from build123d import *

# Parameters (mm, degrees)
SKETCH1_W                      = 330.2
SKETCH1_H                      = 196.85
BOSS_EXTRUDE1_DEPTH            = 11.1125
SKETCH3_W                      = 317.5
SKETCH3_H                      = 184.15
CUT_EXTRUDE1_DEPTH             = 193.533057632
FILLET1_R                      = 6.35
SKETCH4_W                      = 6.35
SKETCH4_H                      = 11.1125
BOSS_EXTRUDE2_DEPTH            = 184.15
FILLET2_R                      = 6.35
F_8_CLEARANCE_HOLE1_REACH      = 346.736
F_8_CLEARANCE_HOLE1_BORE_R     = 2.2479
F_4_40_TAPPED_HOLE1_AT_2_COUNT = 2
F_4_40_TAPPED_HOLE1_AT_2_PITCH = 57.15
F_4_40_TAPPED_HOLE1_AT_3_COUNT = 2
F_4_40_TAPPED_HOLE1_AT_3_PITCH = 117.475
F_4_40_TAPPED_HOLE1_AT_4_COUNT = 2
F_4_40_TAPPED_HOLE1_AT_4_PITCH = 187.325
F_4_40_TAPPED_HOLE1_AT_5_COUNT = 2
F_4_40_TAPPED_HOLE1_AT_5_PITCH = 247.65
F_4_40_TAPPED_HOLE1_AT_6_COUNT = 2
F_4_40_TAPPED_HOLE1_AT_6_PITCH = 317.5
F_4_40_TAPPED_HOLE2_AT_2_COUNT = 2
F_4_40_TAPPED_HOLE2_AT_2_PITCH = 95.25
LPATTERN1_COUNT                = 2
LPATTERN1_PITCH                = 120.015
CUT_EXTRUDE2_REACH             = 346.736
SKETCH13_W                     = 22.225
SKETCH13_H                     = 5.08


with BuildPart() as part:
    # Sketch1 → Boss-Extrude1 (new body)
    with BuildSketch(Plane(origin=(0, 0, 0), x_dir=(1, 0, 0), z_dir=(0, 1, 0))):
        Rectangle(SKETCH1_W, SKETCH1_H)
    extrude(amount=BOSS_EXTRUDE1_DEPTH)

    # Sketch3 → Cut-Extrude1 (cut, through all)
    with BuildSketch(Plane(origin=(0, 11.1125, 0), x_dir=(1, 0, 0), z_dir=(0, 1, 0))):
        Rectangle(SKETCH3_W, SKETCH3_H)
    extrude(amount=-CUT_EXTRUDE1_DEPTH, mode=Mode.SUBTRACT)

    # Fillet1
    fillet1_edges = [part.edges().sort_by_distance(p)[0] for p in [
        (158.75, 5.55625, -92.075),
        (158.75, 5.55625, 92.075),
        (-158.75, 5.55625, 92.075),
        (-158.75, 5.55625, -92.075),
        (165.1, 5.55625, 98.425),
        (-165.1, 5.55625, 98.425),
        (-165.1, 5.55625, -98.425),
        (165.1, 5.55625, -98.425),
    ]]
    fillet(fillet1_edges, radius=FILLET1_R)

    # Sketch4 → Boss-Extrude2 (add)
    with BuildSketch(Plane.XY.offset(-92.075)):
        with Locations((-41.275, 5.55625)):
            Rectangle(SKETCH4_W, SKETCH4_H)
    extrude(amount=BOSS_EXTRUDE2_DEPTH)

    # Fillet2
    fillet2_edges = [part.edges().sort_by_distance(p)[0] for p in [
        (-44.45, 5.55625, -92.075),
        (-38.1, 5.55625, -92.075),
        (-44.45, 5.55625, 92.075),
        (-38.1, 5.55625, 92.075),
    ]]
    fillet(fillet2_edges, radius=FILLET2_R)

    # 8 Clearance Hole1 bore → 8 Clearance Hole1 (cut, up to next)
    with BuildSketch(Plane.ZY.offset(165.1), mode=Mode.PRIVATE) as f_8_clearance_hole1_sk1:
        with Locations((-78.105, 6.0325)):
            Circle(F_8_CLEARANCE_HOLE1_BORE_R)
    f_8_clearance_hole1_tool1 = extrude(f_8_clearance_hole1_sk1.sketch, amount=-F_8_CLEARANCE_HOLE1_REACH, mode=Mode.PRIVATE) & part.part
    # 8 Clearance Hole1 bore → 8 Clearance Hole1 (cut, up to next)
    with BuildSketch(Plane.ZY.offset(165.1), mode=Mode.PRIVATE) as f_8_clearance_hole1_sk2:
        with Locations((0, 6.0325)):
            Circle(F_8_CLEARANCE_HOLE1_BORE_R)
    f_8_clearance_hole1_tool2 = extrude(f_8_clearance_hole1_sk2.sketch, amount=-F_8_CLEARANCE_HOLE1_REACH, mode=Mode.PRIVATE) & part.part
    # 8 Clearance Hole1 bore → 8 Clearance Hole1 (cut, up to next)
    with BuildSketch(Plane.ZY.offset(165.1), mode=Mode.PRIVATE) as f_8_clearance_hole1_sk3:
        with Locations((78.105, 6.0325)):
            Circle(F_8_CLEARANCE_HOLE1_BORE_R)
    f_8_clearance_hole1_tool3 = extrude(f_8_clearance_hole1_sk3.sketch, amount=-F_8_CLEARANCE_HOLE1_REACH, mode=Mode.PRIVATE) & part.part
    f_8_clearance_hole1_1 = f_8_clearance_hole1_tool1.solids().sort_by_distance((-165.1, 6.0325, -78.105))[0]
    add(f_8_clearance_hole1_1, mode=Mode.SUBTRACT)
    f_8_clearance_hole1_2 = f_8_clearance_hole1_tool2.solids().sort_by_distance((-165.1, 6.0325, 0))[0]
    add(f_8_clearance_hole1_2, mode=Mode.SUBTRACT)
    f_8_clearance_hole1_3 = f_8_clearance_hole1_tool3.solids().sort_by_distance((-165.1, 6.0325, 78.105))[0]
    add(f_8_clearance_hole1_3, mode=Mode.SUBTRACT)
    f_8_clearance_hole1 = f_8_clearance_hole1_1 + f_8_clearance_hole1_2 + f_8_clearance_hole1_3  # 8 Clearance Hole1 as one shape, for the pattern or mirror that repeats it

    # Mirror1: 8 Clearance Hole1 across plane
    add(f_8_clearance_hole1.mirror(Plane(origin=(0, 0, 0), x_dir=(0, 0, 1), z_dir=(1, 0, 0))), mode=Mode.SUBTRACT)

    # Sketch9 → 4-40 Tapped Hole1 (revolve, cut)
    with BuildSketch(Plane(origin=(-158.75, 0, 94.615), x_dir=(0, 0, -1), z_dir=(1, 0, 0))):
        Polygon((0, 0), (0, 8.299152758), (1.1303, 7.62), (1.1303, 0), align=None)
    f_4_40_tapped_hole1 = revolve(axis=Axis((-158.75, -6.35, 94.615), (0, 1, 0)), mode=Mode.SUBTRACT)

    # 4-40 Tapped Hole1 at 2: 4-40 Tapped Hole1 ×2
    with Locations(*[(i * F_4_40_TAPPED_HOLE1_AT_2_PITCH, 0, 0) for i in range(1, F_4_40_TAPPED_HOLE1_AT_2_COUNT)]):
        add(f_4_40_tapped_hole1, mode=Mode.SUBTRACT)

    # 4-40 Tapped Hole1 at 3: 4-40 Tapped Hole1 ×2
    with Locations(*[(i * F_4_40_TAPPED_HOLE1_AT_3_PITCH, 0, 0) for i in range(1, F_4_40_TAPPED_HOLE1_AT_3_COUNT)]):
        add(f_4_40_tapped_hole1, mode=Mode.SUBTRACT)

    # 4-40 Tapped Hole1 at 4: 4-40 Tapped Hole1 ×2
    with Locations(*[(i * F_4_40_TAPPED_HOLE1_AT_4_PITCH, 0, 0) for i in range(1, F_4_40_TAPPED_HOLE1_AT_4_COUNT)]):
        add(f_4_40_tapped_hole1, mode=Mode.SUBTRACT)

    # 4-40 Tapped Hole1 at 5: 4-40 Tapped Hole1 ×2
    with Locations(*[(i * F_4_40_TAPPED_HOLE1_AT_5_PITCH, 0, 0) for i in range(1, F_4_40_TAPPED_HOLE1_AT_5_COUNT)]):
        add(f_4_40_tapped_hole1, mode=Mode.SUBTRACT)

    # 4-40 Tapped Hole1 at 6: 4-40 Tapped Hole1 ×2
    with Locations(*[(i * F_4_40_TAPPED_HOLE1_AT_6_PITCH, 0, 0) for i in range(1, F_4_40_TAPPED_HOLE1_AT_6_COUNT)]):
        add(f_4_40_tapped_hole1, mode=Mode.SUBTRACT)

    # Mirror2: 4-40 Tapped Hole1 across plane
    add(f_4_40_tapped_hole1.mirror(Plane.XY), mode=Mode.SUBTRACT)

    # Mirror2 copy 1 sketch → Mirror2 copy 1 (revolve, cut)
    with BuildSketch(Plane(origin=(-101.6, 0, -94.615), x_dir=(0, 0, 1), z_dir=(1, 0, 0))):
        Polygon((0, 0), (0, -8.299152758), (1.1303, -7.62), (1.1303, 0), align=None)
    revolve(axis=Axis((-101.6, -6.35, -94.615), (0, -1, 0)), mode=Mode.SUBTRACT)

    # Mirror2 copy 2 sketch → Mirror2 copy 2 (revolve, cut)
    with BuildSketch(Plane(origin=(-41.275, 0, -94.615), x_dir=(0, 0, 1), z_dir=(1, 0, 0))):
        Polygon((0, 0), (0, -8.299152758), (1.1303, -7.62), (1.1303, 0), align=None)
    revolve(axis=Axis((-41.275, -6.35, -94.615), (0, -1, 0)), mode=Mode.SUBTRACT)

    # Mirror2 copy 3 sketch → Mirror2 copy 3 (revolve, cut)
    with BuildSketch(Plane(origin=(28.575, 0, -94.615), x_dir=(0, 0, 1), z_dir=(1, 0, 0))):
        Polygon((0, 0), (0, -8.299152758), (1.1303, -7.62), (1.1303, 0), align=None)
    revolve(axis=Axis((28.575, -6.35, -94.615), (0, -1, 0)), mode=Mode.SUBTRACT)

    # Mirror2 copy 4 sketch → Mirror2 copy 4 (revolve, cut)
    with BuildSketch(Plane(origin=(88.9, 0, -94.615), x_dir=(0, 0, 1), z_dir=(1, 0, 0))):
        Polygon((0, 0), (0, -8.299152758), (1.1303, -7.62), (1.1303, 0), align=None)
    revolve(axis=Axis((88.9, -6.35, -94.615), (0, -1, 0)), mode=Mode.SUBTRACT)

    # Mirror2 copy 5 sketch → Mirror2 copy 5 (revolve, cut)
    with BuildSketch(Plane(origin=(158.75, 0, -94.615), x_dir=(0, 0, 1), z_dir=(1, 0, 0))):
        Polygon((0, 0), (0, -8.299152758), (1.1303, -7.62), (1.1303, 0), align=None)
    revolve(axis=Axis((158.75, -6.35, -94.615), (0, -1, 0)), mode=Mode.SUBTRACT)

    # Sketch11 → 4-40 Tapped Hole2 (revolve, cut)
    with BuildSketch(Plane(origin=(-161.29, 0, 47.625), x_dir=(0, 0, -1), z_dir=(1, 0, 0))):
        Polygon((0, 0), (0, 8.299152758), (1.1303, 7.62), (1.1303, 0), align=None)
    f_4_40_tapped_hole2 = revolve(axis=Axis((-161.29, -6.35, 47.625), (0, 1, 0)), mode=Mode.SUBTRACT)

    # 4-40 Tapped Hole2 at 2: 4-40 Tapped Hole2 ×2
    with Locations(*[(0, 0, -i * F_4_40_TAPPED_HOLE2_AT_2_PITCH) for i in range(1, F_4_40_TAPPED_HOLE2_AT_2_COUNT)]):
        add(f_4_40_tapped_hole2, mode=Mode.SUBTRACT)

    # LPattern1: 4-40 Tapped Hole2 ×2
    with Locations(*[(i * LPATTERN1_PITCH, 0, 0) for i in range(1, LPATTERN1_COUNT)]):
        add(f_4_40_tapped_hole2, mode=Mode.SUBTRACT)

    # LPattern1 copy 1 sketch → LPattern1 copy 1 (revolve, cut)
    with BuildSketch(Plane(origin=(-41.275, 0, -47.625), x_dir=(0, 0, -1), z_dir=(1, 0, 0))):
        Polygon((0, 0), (0, 8.299152758), (1.1303, 7.62), (1.1303, 0), align=None)
    revolve(axis=Axis((-41.275, -6.35, -47.625), (0, 1, 0)), mode=Mode.SUBTRACT)

    # Mirror3: 4-40 Tapped Hole2 across plane
    add(f_4_40_tapped_hole2.mirror(Plane(origin=(0, 0, 0), x_dir=(0, 0, 1), z_dir=(1, 0, 0))), mode=Mode.SUBTRACT)

    # Mirror3 copy 1 sketch → Mirror3 copy 1 (revolve, cut)
    with BuildSketch(Plane(origin=(161.29, 0, -47.625), x_dir=(0, 0, -1), z_dir=(-1, 0, 0))):
        Polygon((0, 0), (0, -8.299152758), (1.1303, -7.62), (1.1303, 0), align=None)
    revolve(axis=Axis((161.29, -6.35, -47.625), (0, -1, 0)), mode=Mode.SUBTRACT)

    # Sketch13 → Cut-Extrude2 (cut, up to next)
    with BuildSketch(Plane(origin=(165.1, 0, 0), x_dir=(0, 0, -1), z_dir=(1, 0, 0)), mode=Mode.PRIVATE) as cut_extrude2_sk1:
        with Locations((33.3375, 8.5725)):
            Rectangle(SKETCH13_W, SKETCH13_H)
    cut_extrude2_tool1 = extrude(cut_extrude2_sk1.sketch, amount=-CUT_EXTRUDE2_REACH, mode=Mode.PRIVATE) & part.part
    add(cut_extrude2_tool1.solids().sort_by_distance((165.1, 8.5725, -33.3375))[0], mode=Mode.SUBTRACT)


solid = part.part
Input: part model. Units: mm. Frame: model coordinates. A direction names the side the tool comes from. Give positions to 0.01 mm unless a question says otherwise; leave off trailing zeros. Loops run counter-clockwise (first coordinate to the right, second up) from the corner with the lowest first, then second, coordinate; pieces in that order, holes last. Notation, with made-up numbers: (56, 29) -> (100, 29) arc R27 cw to (100, 55) -> close; hole circle Ø7 at (24, 18.25). An arc over 180 degrees is marked (long way). Answer as a JSON object with one key per item and string values. Group by question number.
Item 1: Cut plane A-A, the plane z = 36. Return the cut outline in (x, y).
Item 2: Reachability of faces 1 (the flat face through (162, 6.032, -33)), 2 (the cylindrical face through (156.84, 5.478, 90.264)), 3 (the flat face through (-50, 0, -95)) from +Z, -Z, +X, -X, +Y, -Y: full face, straight path, thin tool, end or side. Return the list, or none.
Item 3: Line query: probe 1 along X at (y, z) = (7, -8); probe 2 along X at (y, z) = (5.25, -86.5); probe 3 along Z at (x, y) = (-41, 7.5) (3 decimals). Output: solid intervals per line, ascending.
Item 4: Cut plane B-B, the plane x = -8. Return the cut outline in (y, z) (1 decimal).
Item 5: Pull-direction query (Z, two-part tool) for faces 4 (the flat face through (-44.45, 5, -1)), 5 (the flat face through (-2, 5, 98.425)), 6 (the flat face through (-50, 11.112, 94)); classes: released by +Z, released by -Z, zero draft, split by the parting line, or undercut.
Item 6: Pin query (flat end, axial travel): P1, Ø2.5, axis at y = 6.03, z = 0, coming from the -X side; P2, Ø2, axis at x = -101.6, z = 94.615, coming from the -Y side; P3, Ø1.4, axis at x = 158.75, z = -94.615, coming from the -Y side. Return the tip coordinate at first contact, or that it passes through.
Checks:
{
 "1": {"outline": "(-165.1, 0) -> (-158.75, 0) -> (-158.75, 11.11) -> (-165.1, 11.11) -> close; (-44.45, 0) -> (-38.1, 0) -> (-38.1, 11.11) -> (-44.45, 11.11) -> close; (158.75, 0) -> (165.1, 0) -> (165.1, 11.11) -> (158.75, 11.11) -> close"},
 "2": {"face 1": "+X, +Y", "face 2": "+Y, -Y", "face 3": "+Z, -Z, +X, -X, -Y"},
 "3": {"probe 1": "x = -165.1 to -158.75, -44.45 to -38.1, 158.75 to 165.1", "probe 2": "x = -165.1 to -158.7, -44.5 to -38.05, 158.7 to 165.1", "probe 3": "z = -98.425 to -95.711, -93.519 to -48.721, -46.529 to 46.529, 48.721 to 93.519, 95.711 to 98.425"},
 "4": {"outline": "(0, -98.4) -> (11.1, -98.4) -> (11.1, -92.1) -> (0, -92.1) -> close; (0, 92.1) -> (11.1, 92.1) -> (11.1, 98.4) -> (0, 98.4) -> close"},
 "5": {"face 4": "undercut", "face 5": "released by +Z", "face 6": "zero draft"},
 "6": {"P1": "stops at x = -44.45", "P2": "stops at y = 7.7", "P3": "stops at y = 7.88"}
}
